Autodesk Inventor part; units mm, degrees
ref_plane "YZ Plane" through (0, 0, 0) normal (1, 0, 0) x (0, 1, 0)
ref_plane "XZ Plane" through (0, 0, 0) normal (0, 1, 0) x (-1, 0, 0)
ref_plane "XY Plane" through (0, 0, 0) normal (0, 0, 1) x (1, 0, 0)
sketch "Sketch1" plane through (0, 0, 0) normal (1, 0, 0) x (0, 1, 0)
  line L0 (47.75, -10) -> (-47.75, -10)
  line L1 (-47.75, -10) -> (-47.75, 10)
  line L2 (-47.75, 10) -> (47.75, 10)
  line L3 (47.75, 10) -> (47.75, -10)
  line L4 (47.75, -10) -> (-47.75, 10) construction
  line L5 (-47.75, -10) -> (47.75, 10) construction
  circle A0 centre (40.75, 0) radius 2
  circle A1 centre (-4.25, 0) radius 2
  line L6 (18.25, 25.1028) -> (18.25, -34.7635) construction
  line L7 (-1.75, 23.8417) -> (-1.75, -36.7999) construction
  circle A2 centre (20.75, 0) radius 2
  circle A3 centre (-24.25, 0) radius 2
  line L8 (-41.75, 23.8417) -> (-41.75, -30.9921) construction
  circle A4 centre (34.0833, 0) radius 2
  circle A5 centre (27.4167, 0) radius 2
  circle A6 centre (-10.9167, 0) radius 2
  circle A7 centre (-17.5833, 0) radius 2
  point P0 (0, 0)
  dimension "d1" = 20
  dimension "d4" = 4
  dimension "d5" = 7
  dimension "d6" = 45
  dimension "d7" = 22.5
  dimension "d8" = 20
  dimension "d9" = 22.5
  dimension "d10" = 22.5
  dimension "d11" = 60
  dimension "d18" = 6.6667
  dimension "d25" = 6.6667
  dimension "d30" = 6
extrude "Extrusion1" add sketch "Sketch1" along normal blind 4
sketch "Sketch2" plane through (0, 0, 0) normal (1, 0, 0) x (0, 1, 0)
  line L0 (-41.75, 22.3574) -> (-41.75, -36.9148) construction
  circle A0 centre (-17.5833, 0) radius 2
  circle A1 centre (-10.9167, 0) radius 2
  circle A2 centre (27.4167, 0) radius 2
  circle A3 centre (34.0833, 0) radius 2
  circle A4 centre (-24.25, 0) radius 2
  circle A5 centre (20.75, 0) radius 2
  circle A6 centre (-4.25, 0) radius 2
  circle A7 centre (40.75, 0) radius 2
  line L1 (-47.75, -10) -> (47.75, -10)
  line L2 (47.75, -10) -> (47.75, 10)
  line L3 (47.75, 10) -> (-47.75, 10)
  line L4 (-47.75, 10) -> (-47.75, -10)
  line L5 (47.75, 0) -> (-47.75, 0) construction
  line L6 (-47.75, -10) -> (-47.75, 10)
  line L7 (-59.75, -6.125) -> (-36.75, -6.125)
  line L8 (-36.75, -6.125) -> (-36.75, 6.125)
  line L9 (-36.75, 6.125) -> (-59.75, 6.125)
  line L10 (-59.75, 6.125) -> (-59.75, -6.125)
  line L11 (-59.75, -6.125) -> (-36.75, 6.125) construction
  line L12 (-36.75, -6.125) -> (-59.75, 6.125) construction
  line L13 (-47.75, -10) -> (-63.625, -10)
  line L14 (-63.625, -10) -> (-63.625, 10)
  line L15 (-63.625, 10) -> (-47.75, 10)
  line L16 (-47.75, 10) -> (-47.75, -10)
  line L17 (-32.875, -10) -> (-32.875, 10)
  point P0 (0, 0)
  point P1 (-48.25, 0)
  dimension "d33" = 6
  dimension "d34" = 12.25
  dimension "d35" = 23
  dimension "d36" = 5
  dimension "d37" = 3.875
  dimension "d38" = 3.875
  dimension "d39" = 3.875
extrude "Extrusion2" cut sketch "Sketch2" along normal blind 20 contours L7 L10 L9 L4 | L4 L9 L8 L7
sketch "Sketch3" plane through (0, 0, 0) normal (-1, 0, 0) x (0, 0, 1)
  line L0 (-10, -47.75) -> (-6.125, -47.75)
  line L1 (-10, -47.75) -> (-6.125, -47.75)
  line L2 (6.125, -47.75) -> (10, -47.75)
  line L3 (10, -47.75) -> (6.125, -47.75)
  line L4 (6.125, -36.75) -> (6.125, -47.75)
  line L5 (6.125, -47.75) -> (10, -47.75)
  line L6 (10, -47.75) -> (10, 47.75)
  line L7 (10, 47.75) -> (-10, 47.75)
  line L8 (-10, 47.75) -> (-10, -47.75)
  line L9 (-10, -47.75) -> (-6.125, -47.75)
  line L10 (-6.125, -47.75) -> (-6.125, -36.75)
  line L11 (-6.125, -36.75) -> (6.125, -36.75)
  circle A0 centre (0, -17.5833) radius 2
  circle A1 centre (0, -10.9167) radius 2
  circle A2 centre (0, 27.4167) radius 2
  circle A3 centre (0, 34.0833) radius 2
  circle A4 centre (0, -24.25) radius 2
  circle A5 centre (0, 20.75) radius 2
  circle A6 centre (0, -4.25) radius 2
  circle A7 centre (0, 40.75) radius 2
  line L12 (-6.125, -36.75) -> (6.125, -36.75)
  line L13 (6.125, -36.75) -> (6.125, -59.75)
  line L14 (6.125, -59.75) -> (-6.125, -59.75)
  line L15 (-6.125, -59.75) -> (-6.125, -36.75)
  line L16 (-10, 47.75) -> (-10, -47.75)
  line L17 (-10, -32.875) -> (10, -32.875)
  line L18 (10, -32.875) -> (10, -63.625)
  line L19 (10, -63.625) -> (-10, -63.625)
  line L20 (-10, -63.625) -> (-10, -32.875)
  point P0 (0, 0)
  dimension "d44" = 23
  dimension "d45" = 3.875
  dimension "d46" = 3.875
  dimension "d47" = 3.875
extrude "Extrusion4" add sketch "Sketch3" along normal blind 20 contours L8 L17 L6 L2 L4 L11 L10 L0 | L0 L15 L14 L13 L2 L18 L19 L20
sketch "Sketch5" plane through (0, 0, 0) normal (1, 0, 0) x (0, 0, -1)
  line L0 (-6.125, -47.75) -> (-10, -47.75)
  line L1 (-10, -63.625) -> (-10, -47.75)
  line L2 (10, -63.625) -> (-10, -63.625)
  line L3 (10, -47.75) -> (10, -63.625)
  line L4 (10, -47.75) -> (6.125, -47.75)
  line L5 (6.125, -47.75) -> (6.125, -59.75)
  line L6 (6.125, -59.75) -> (-6.125, -59.75)
  line L7 (-6.125, -59.75) -> (-6.125, -47.75)
  point P0 (0, 0)
extrude "Extrusion5" add sketch "Sketch5" along normal blind 4
sketch "Sketch6" plane through (0, 0, 0) normal (-1, 0, 0) x (0, 0, 1)
  line L0 (-10, -32.875) -> (10, -32.875)
  line L1 (10, -32.875) -> (10, 47.75)
  line L2 (10, 47.75) -> (-10, 47.75)
  line L3 (-10, 47.75) -> (-10, -32.875)
  circle A0 centre (0, -17.5833) radius 2
  circle A1 centre (0, -10.9167) radius 2
  circle A2 centre (0, 27.4167) radius 2
  circle A3 centre (0, 34.0833) radius 2
  circle A4 centre (0, -24.25) radius 2
  circle A5 centre (0, 20.75) radius 2
  circle A6 centre (0, -4.25) radius 2
  circle A7 centre (0, 40.75) radius 2
  circle A8 centre (0, -30.375) radius 0.875
  point P0 (0, 0)
  dimension "d52" = 2.5
  dimension "d53" = 1.75
extrude "Extrusion6" cut sketch "Sketch6" against normal blind 4 contours A8
sketch "Sketch7" plane through (0, 47.75, 10) normal (0, 0, 1) x (1, 0, 0)
  line L0 (4, 0) -> (4, -111.375)
  line L1 (0, 0) -> (4, 0)
  line L2 (0, -80.625) -> (0, 0)
  line L3 (0, -80.625) -> (-20, -80.625)
  line L4 (-20, -111.375) -> (-20, -80.625)
  line L5 (4, -111.375) -> (-20, -111.375)
  line L6 (4, -84.5) -> (4, -107.5)
  line L7 (-20, -84.5) -> (4, -84.5)
  line L8 (-20, -107.5) -> (-20, -84.5)
  line L9 (4, -107.5) -> (-20, -107.5)
  line L10 (-16.125, -88.375) -> (0.125, -88.375)
  line L11 (0.125, -88.375) -> (0.125, -103.625)
  line L12 (0.125, -103.625) -> (-16.125, -103.625)
  line L13 (-16.125, -103.625) -> (-16.125, -88.375)
  point P0 (0, -47.75)
  dimension "d56" = 3.875
  dimension "d57" = 3.875
  dimension "d58" = 3.875
  dimension "d59" = 3.875
extrude "Extrusion7" cut sketch "Sketch7" against normal blind 20 contours L10 L11 L12 L13
sketch "Sketch8" plane through (4, 47.75, -10) normal (0, 0, -1) x (-1, 0, 0)
  line L0 (24, -84.5) -> (0, -84.5)
  line L1 (20.125, -88.375) -> (20.125, -103.625)
  line L2 (20.125, -103.625) -> (3.875, -103.625)
  line L3 (3.875, -103.625) -> (3.875, -88.375)
  line L4 (3.875, -88.375) -> (20.125, -88.375)
  line L5 (4, 0) -> (4, -80.625)
  line L6 (4, 0) -> (0, 0)
  line L7 (0, -111.375) -> (0, 0)
  line L8 (0, -111.375) -> (24, -111.375)
  line L9 (24, -80.625) -> (24, -111.375)
  line L10 (4, -80.625) -> (24, -80.625)
  line L11 (4, -80.625) -> (4, 0)
  line L12 (4, 0) -> (4, -80.625)
  line L13 (24, -80.625) -> (4, 0)
  point P0 (4, -47.75)
extrude "Extrusion8" add sketch "Sketch8" against normal blind 3 contours L10 L5 L13
mirror "Mirror2" about plane through (0, 0, 0) normal (0, 0, 1) of "Extrusion8"
sketch "Sketch9" plane through (4, 0, 0) normal (1, 0, 0) x (0, 0, -1)
  circle A0 centre (0, -30.375) radius 0.875
  line L0 (10, -63.625) -> (10, 47.75)
  line L1 (10, 47.75) -> (-10, 47.75)
  line L2 (-10, 47.75) -> (-10, -63.625)
  line L3 (-10, -63.625) -> (10, -63.625)
  line L4 (6.125, -36.75) -> (6.125, -59.75)
  line L5 (6.125, -59.75) -> (-6.125, -59.75)
  line L6 (-6.125, -59.75) -> (-6.125, -36.75)
  line L7 (-6.125, -36.75) -> (6.125, -36.75)
  circle A1 centre (0, 40.75) radius 2
  circle A2 centre (0, -4.25) radius 2
  circle A3 centre (0, 20.75) radius 2
  circle A4 centre (0, -24.25) radius 2
  circle A5 centre (0, 34.0833) radius 2
  circle A6 centre (0, 27.4167) radius 2
  circle A7 centre (0, -10.9167) radius 2
  circle A8 centre (0, -17.5833) radius 2
  point P0 (0, 0)
properties part number "TopRearLeg"
Could you check a few things on this model? Use its own coordinates, in mm. A direction names the side the tool comes from. Coordinates: 2 decimals unless noted, no trailing zeros. Order: outer loops, then holes, each group sorted by start corner. A loop starts at its lowest first (then second) coordinate and runs counter-clockwise, first axis right, second up. Notation, with made-up numbers: M 27,32 L 76,32 A8 ccw 76,44 Z; hole C 47,45 d2. An arc over 180 degrees is marked long. Use one line per item in the form item = value. Start each with the question number.
1. We'd pull the mould along Y, two halves only. Please class faces 4 (the flat face through (-8, -36.75, 0)), 5 (the flat face through (-8, -63.625, 0)), 6 (the flat face through (4, -7, 0)): +Y half, -Y half, draft (parallel to the pull), parting line (faces both ways), or undercut.
2. For pin 1 (4.5 mm diameter, centred on y = 40.75, z = 0, fed in from -X); pin 2 (4 mm diameter, centred on x = -15.5, z = 0.5, fed in from +Y) (3 decimals); pin 3 (11 mm diameter, centred on y = 18, z = 3, fed in from -X), each with a flat end and sliding along its axis, tell me the tip position at first contact or that it passes through.
3. Suppose I cut it at C-C on x = -9.25. Write out the boundary of the cut face in (y, z) (3 decimals).
4. Please list where these lines run through material, in increasing order: line 1 (Z direction, x = 1.6, y = -4.25); line 2 (Z direction, x = -18, y = -42) (3 decimals); line 3 (Y direction, x = -12.25, z = -2.25) (3 decimals).
5. Suppose I cut it at D-D on y = -4.25. Write out the boundary of the cut face in (x, z), then the cut area to 3 significant figures.
6. Suppose I cut it at A-A on y = -51. Write out the boundary of the cut face in (x, z) (3 decimals).
7. Suppose I cut it at B-B on z = 3.5. Write out the boundary of the cut face in (x, y) (3 decimals), then the cut area to 4 significant figures.
8. On a 3-axis mill with a long thin cutter (end or side, diameter ignored), from which of +Z, -Z, +X, -X, +Y, -Y can I reach the whole of each face in a straight line? I mean faces 1 (the flat face through (0, 7, 0)), 2 (the flat face through (-8, -59.75, 0)), 3 (the flat face through (-8, -55.875, 8)). Say none if no direction works.
Geometry says:
q1.face_4 = undercut
q1.face_5 = -Y half
q1.face_6 = draft
q2.pin_1 = 0
q2.pin_2 = -32.875
q2.pin_3 = -8.32
q3.outline = M -63.625,-10 L -55.875,-10 L -55.875,-6.125 L -59.75,-6.125 L -59.75,6.125 L -55.875,6.125 L -55.875,10 L -63.625,10 Z; M -40.625,-10 L 10.461,-10 L 10.461,-7 L -32.875,-7 L -32.875,7 L 10.461,7 L 10.461,10 L -40.625,10 L -40.625,6.125 L -36.75,6.125 L -36.75,-6.125 L -40.625,-6.125 Z
q4.line_1 = -10 to -2, 2 to 10
q4.line_2 = -10 to -6.125, 6.125 to 10
q4.line_3 = -63.625 to -59.75, -36.75 to -32.875
q5.outline = M -12.9,-10 L 4,-10 L 4,-2 L 0,-2 L 0,-7 L -12.9,-7 Z; M -12.9,7 L 0,7 L 0,2 L 4,2 L 4,10 L -12.9,10 Z
q5.area = 141 mm^2
q6.outline = M -20,-10 L -16.125,-10 L -16.125,-6.125 L -20,-6.125 Z; M -20,6.125 L -16.125,6.125 L -16.125,10 L -20,10 Z; M 0.125,-10 L 4,-10 L 4,-6.125 L 0.125,-6.125 Z; M 0.125,6.125 L 4,6.125 L 4,10 L 0.125,10 Z
q7.outline = M -20,-63.625 L 4,-63.625 L 4,-59.75 L -20,-59.75 Z; M -20,-36.75 L 4,-36.75 L 4,47.75 L 0,47.75 L 0,-32.875 L -20,-32.875 Z
q7.area = 508.5 mm^2
q8.face_1 = -X, +Y
q8.face_2 = +X, -X
q8.face_3 = +Z, -Z
